```python
from build123d import *

# Parameters (mm, degrees)
F1_DEPTH = 25.4
F0_W     = 1295.4
F0_H     = 38.1
F0_W_2   = 152.4
F2_DEPTH = 660.4
F0_W_3   = 381
F0_H_2   = 6.35
F3_DEPTH = 50.8


with BuildPart() as f1:
    # F0 (on Top) → F1 (new body)
    with BuildSketch(Plane.XY):
        with BuildLine():
            Line((722.1747212052, 300.0245658736), (569.7747212052, 300.0245658736))
            Line((569.7747212052, 300.0245658736), (569.7747212052, 274.6245658736))
            ThreePointArc((569.7747212052, 274.6245658736), (596.7154895684, 263.4653342368), (607.8747212052, 236.5245658736))
            Line((607.8747212052, 236.5245658736), (722.1747212052, 236.5245658736))
            Line((722.1747212052, 236.5245658736), (722.1747212052, 300.0245658736))
        make_face()
        with BuildLine():
            Line((569.7747212052, 300.0245658736), (-725.6252787948, 300.0245658736))
            Line((-725.6252787948, 300.0245658736), (-725.6252787948, -265.1254341264))
            Line((-725.6252787948, -265.1254341264), (-344.6252787948, -265.1254341264))
            Line((-344.6252787948, -265.1254341264), (-344.6252787948, -271.4754341264))
            Line((-344.6252787948, -271.4754341264), (722.1747212052, -271.4754341264))
            Line((722.1747212052, -271.4754341264), (722.1747212052, 236.5245658736))
            Line((722.1747212052, 236.5245658736), (607.8747212052, 236.5245658736))
            ThreePointArc((607.8747212052, 236.5245658736), (542.833952842, 209.5837975104), (569.7747212052, 274.6245658736))
            Line((569.7747212052, 274.6245658736), (569.7747212052, 300.0245658736))
        make_face()
    extrude(amount=-F1_DEPTH)

    # F0 (on Top) → F2 (join)
    with BuildSketch(Plane.XY):
        with Locations((-77.9252787948, 319.0745658736)):
            Rectangle(F0_W, F0_H)
        with Locations((645.9747212052, 319.0745658736)):
            Rectangle(F0_W_2, F0_H)
        Polygon((760.2747212052, 338.1245658736), (722.1747212052, 338.1245658736), (722.1747212052, 300.0245658736), (722.1747212052, 236.5245658736), (722.1747212052, -271.4754341264), (760.2747212052, -271.4754341264), align=None)
        Polygon((-725.6252787948, 338.1245658736), (-763.7252787948, 338.1245658736), (-763.7252787948, -271.4754341264), (-725.6252787948, -271.4754341264), (-725.6252787948, -265.1254341264), (-725.6252787948, 300.0245658736), align=None)
    extrude(amount=-F2_DEPTH)

    # F0 (on Top) → F3 (join)
    with BuildSketch(Plane.XY):
        with Locations((-535.1252787948, -268.3004341264)):
            Rectangle(F0_W_3, F0_H_2)
    extrude(amount=-F3_DEPTH)


solid = f1.part
```
Source: CAD feature listing. Evaluate the final solid. Frame: model axes, mm. A direction names the side the tool comes from. Give positions to 0.01 mm unless a question says otherwise; leave off trailing zeros. Write each loop counter-clockwise with the first axis right and the second up, starting at its lowest first coordinate (ties: lowest second). Pieces come first, ordered by that corner, then holes. Notation, with made-up numbers: (88.25, 36.25) - (109.25, 36.25) arc R25 cw to (109.25, 66.25) - close; hole circle Ø1 at (57.25, 6). An arc over 180 degrees is marked (long way). One line per item, written item: value. Start each with the question number.
Q1. First-contact query: pin 1 Ø6 at (x, z) = (-396, -459) entering from -Y; pin 2 Ø1.5 at (x, y) = (-239.5, 213.5) entering from -Z; pin 3 Ø1.9 at (x, y) = (-482, -268.5) entering from -Z. Flat tips, straight axial feed; report the tip coordinate or a pass-through.
Q2. Material intervals for probe 1 along X at (y, z) = (124, -328.5); probe 2 along Z at (x, y) = (-154.5, 268.5); probe 3 along Y at (x, z) = (-631, -456.5), sorted ascending. Write a range as from..to.
Q3. Set-up query: faces 5 (the face through (722.175, 18, -338)), 6 (the face through (-62, -271.475, -11)). Return all of +Z, -Z, +X, -X, +Y, -Y with unobstructed straight access to the full face (end or side cutting, diameter ignored); none if empty.
Q4. Section query C-C, the plane y = 252.5. Return the cut outline in (x, z).
Q5. Draft query along X for faces 1 (the face through (541.693, 210.775, -12.522)), 2 (the face through (-763.725, 38, -326)), 3 (the face through (760.275, 29, -326)), 4 (the face through (-62, 306, -660.4)). Return one class per face: +X half, -X half, draft (parallel to the pull), parting line (faces both ways), or undercut.
Q6. Section query D-D, the plane x = -134.5. Return the cut outline in (y, z), then the cut area to 3 significant figures.
Q7. Section query A-A, the plane x = -412. Return the cut outline in (y, z), then the cut area to 3 significant figures.
Q8. Section query B-B, the plane z = -467. Return the cut outline in (x, y), then the cut area to 3 significant figures.
Answer:
1. pin 1: stops at y = 300.02
1. pin 2: stops at z = -25.4
1. pin 3: stops at z = -50.8
2. probe 1: x = -763.73..-725.63, 722.17..760.27
2. probe 2: z = -25.4..0
2. probe 3: y = 300.02..338.12
3. face 5: -Z, -Y
3. face 6: +Z, -Z, +X, -X, -Y
4. outline: (-763.73, -660.4) - (-725.63, -660.4) - (-725.63, -25.4) - (535.19, -25.4) - (535.19, 0) - (-763.73, 0) - close; (604.36, -25.4) - (722.17, -25.4) - (722.17, -660.4) - (760.27, -660.4) - (760.27, 0) - (604.36, 0) - close
5. face 1: undercut
5. face 2: -X half
5. face 3: +X half
5. face 4: draft
6. outline: (-271.48, -25.4) - (300.02, -25.4) - (300.02, -660.4) - (338.12, -660.4) - (338.12, 0) - (-271.48, 0) - close
6. area: 39,700 mm2
7. outline: (-271.48, -50.8) - (-265.13, -50.8) - (-265.13, -25.4) - (300.02, -25.4) - (300.02, -660.4) - (338.12, -660.4) - (338.12, 0) - (-271.48, 0) - close
7. area: 39,800 mm2
8. outline: (-763.73, -271.48) - (-725.63, -271.48) - (-725.63, 300.02) - (722.17, 300.02) - (722.17, -271.48) - (760.27, -271.48) - (760.27, 338.12) - (-763.73, 338.12) - close
8. area: 102,000 mm2
